from build123d import *

# Parameters (mm, degrees)
F1_DEPTH       = 40
F2_START       = 34
F2_DEPTH       = 6
F3_DEPTH       = 6
F5_D           = 5
F5_DEPTH       = 8
F5_CSINK_D     = 6
F5_CSINK_ANGLE = 90
F5_TIP         = 1.5021515476
F7_D           = 10
F8_D           = 5
F9_SIZE        = 4
F11_D          = 10
F12_R          = 10
F13_D          = 5
F15_D          = 5
F15_DEPTH      = 12
F15_TIP        = 1.5021515476
F16_START      = -7
F14_R          = 5.5
F16_DEPTH      = 5
F17_DEPTH      = 3


with BuildPart() as f1:
    # F0 (on Top) → F1 (new body)
    with BuildSketch(Plane.XY):
        with BuildLine():
            Line((-8.2927711273, 81.5647094006), (-7.3107365454, 75.6475586596))
            ThreePointArc((-7.3107365454, 75.6475586596), (-6.1560843706, 75.7502648525), (-5, 75.8353479586))
            Line((-5, 75.8353479586), (-5, 81.8325844183))
            ThreePointArc((-5, 81.8325844183), (-6.6477349765, 81.7152341505), (-8.2927711273, 81.5647094006))
        make_face()
        with BuildLine():
            Line((-5, 81.8325844183), (-5, 75.8353479586))
            ThreePointArc((-5, 75.8353479586), (0, 76), (5, 75.8353479586))
            Line((5, 75.8353479586), (5, 100.8353479586))
            Line((5, 100.8353479586), (-5, 100.8353479586))
            Line((-5, 100.8353479586), (-5, 81.8325844183))
        make_face()
        with BuildLine():
            ThreePointArc((-13, 68.7822651561), (44.6654228683, 53.8980519128), (70, 0))
            ThreePointArc((70, 0), (44.6654228683, -53.8980519128), (-13, -68.7822651561))
            Line((-13, -68.7822651561), (-13, -74.8799038461))
            ThreePointArc((-13, -74.8799038461), (0, -76), (13, -74.8799038461))
            ThreePointArc((13, -74.8799038461), (18.0414231151, -73.8275494107), (23, -72.4361788059))
            ThreePointArc((23, -72.4361788059), (61.3351449008, -44.8776113446), (76, 0))
            ThreePointArc((76, 0), (55.4797260267, 51.9422756529), (5, 75.8353479586))
            ThreePointArc((5, 75.8353479586), (0, 76), (-5, 75.8353479586))
            ThreePointArc((-5, 75.8353479586), (-6.1560843706, 75.7502648525), (-7.3107365454, 75.6475586596))
            ThreePointArc((-7.3107365454, 75.6475586596), (-9.056731807, 71.7723085764), (-13, 70.1858979679))
            Line((-13, 70.1858979679), (-13, 68.7822651561))
        make_face()
        with BuildLine():
            ThreePointArc((13, -74.8799038461), (0, -76), (-13, -74.8799038461))
            Line((-13, -74.8799038461), (-13, -80.8799038461))
            Line((-13, -80.8799038461), (13, -80.8799038461))
            Line((13, -80.8799038461), (13, -74.8799038461))
        make_face()
        with BuildLine():
            ThreePointArc((23, -72.4361788059), (18.0414231151, -73.8275494107), (13, -74.8799038461))
            Line((13, -74.8799038461), (13, -80.8799038461))
            Line((13, -80.8799038461), (13, -126.8799038461))
            Line((13, -126.8799038461), (23, -126.8799038461))
            Line((23, -126.8799038461), (23, -72.4361788059))
        make_face()
    extrude(amount=F1_DEPTH)

    # F0 (on Top) → F2 (join)
    with BuildSketch(Plane.XY.offset(F2_START)):
        with BuildLine():
            ThreePointArc((-8.009195615, 75.576800578), (-7.6600477823, 75.6129861067), (-7.3107365454, 75.6475586596))
            Line((-7.3107365454, 75.6475586596), (-8.2927711273, 81.5647094006))
            ThreePointArc((-8.2927711273, 81.5647094006), (-11.0489742273, 81.2372577153), (-13.7925136268, 80.8166965449))
            ThreePointArc((-13.7925136268, 80.8166965449), (-9.7567430054, 79.6853320831), (-8, 75.8799038461))
            ThreePointArc((-8, 75.8799038461), (-8.0022994325, 75.7282824834), (-8.009195615, 75.576800578))
        make_face()
        with BuildLine():
            Line((-13, 74.8799038461), (-13, 70.8799038461))
            ThreePointArc((-13, 70.8799038461), (-9.5733045321, 72.2387833907), (-8.009195615, 75.576800578))
            ThreePointArc((-8.009195615, 75.576800578), (-10.5103754149, 75.2697283683), (-13, 74.8799038461))
        make_face()
        with BuildLine():
            ThreePointArc((-17.6052855561, 73.9327662169), (-15.7626356848, 71.7124293023), (-13, 70.8799038461))
            Line((-13, 70.8799038461), (-13, 74.8799038461))
            ThreePointArc((-13, 74.8799038461), (-15.3099687594, 74.441956292), (-17.6052855561, 73.9327662169))
        make_face()
        with BuildLine():
            ThreePointArc((-13.8960239837, 80.7989628029), (-17.3991209977, 78.2564001006), (-17.6052855561, 73.9327662169))
            ThreePointArc((-17.6052855561, 73.9327662169), (-15.3099687594, 74.441956292), (-13, 74.8799038461))
            ThreePointArc((-13, 74.8799038461), (-10.5103754149, 75.2697283683), (-8.009195615, 75.576800578))
            ThreePointArc((-8.009195615, 75.576800578), (-8.0022994325, 75.7282824834), (-8, 75.8799038461))
            ThreePointArc((-8, 75.8799038461), (-9.7567430054, 79.6853320831), (-13.7925136268, 80.8166965449))
            ThreePointArc((-13.7925136268, 80.8166965449), (-13.8442716447, 80.8078462478), (-13.8960239837, 80.7989628029))
        make_face()
        with BuildLine():
            Line((-13, 70.8799038461), (-13, 70.1858979679))
            ThreePointArc((-13, 70.1858979679), (-9.056731807, 71.7723085764), (-7.3107365454, 75.6475586596))
            ThreePointArc((-7.3107365454, 75.6475586596), (-7.6600477823, 75.6129861067), (-8.009195615, 75.576800578))
            ThreePointArc((-8.009195615, 75.576800578), (-9.5733045321, 72.2387833907), (-13, 70.8799038461))
        make_face()
    extrude(amount=F2_DEPTH)

    # F0 (on Top) → F3 (join)
    with BuildSketch(Plane.XY):
        with BuildLine():
            ThreePointArc((-8.009195615, 75.576800578), (-7.6600477823, 75.6129861067), (-7.3107365454, 75.6475586596))
            Line((-7.3107365454, 75.6475586596), (-8.2927711273, 81.5647094006))
            ThreePointArc((-8.2927711273, 81.5647094006), (-11.0489742273, 81.2372577153), (-13.7925136268, 80.8166965449))
            ThreePointArc((-13.7925136268, 80.8166965449), (-9.7567430054, 79.6853320831), (-8, 75.8799038461))
            ThreePointArc((-8, 75.8799038461), (-8.0022994325, 75.7282824834), (-8.009195615, 75.576800578))
        make_face()
        with BuildLine():
            Line((-13, 74.8799038461), (-13, 70.8799038461))
            ThreePointArc((-13, 70.8799038461), (-9.5733045321, 72.2387833907), (-8.009195615, 75.576800578))
            ThreePointArc((-8.009195615, 75.576800578), (-10.5103754149, 75.2697283683), (-13, 74.8799038461))
        make_face()
        with BuildLine():
            ThreePointArc((-17.6052855561, 73.9327662169), (-15.7626356848, 71.7124293023), (-13, 70.8799038461))
            Line((-13, 70.8799038461), (-13, 74.8799038461))
            ThreePointArc((-13, 74.8799038461), (-15.3099687594, 74.441956292), (-17.6052855561, 73.9327662169))
        make_face()
        with BuildLine():
            ThreePointArc((-13.8960239837, 80.7989628029), (-17.3991209977, 78.2564001006), (-17.6052855561, 73.9327662169))
            ThreePointArc((-17.6052855561, 73.9327662169), (-15.3099687594, 74.441956292), (-13, 74.8799038461))
            ThreePointArc((-13, 74.8799038461), (-10.5103754149, 75.2697283683), (-8.009195615, 75.576800578))
            ThreePointArc((-8.009195615, 75.576800578), (-8.0022994325, 75.7282824834), (-8, 75.8799038461))
            ThreePointArc((-8, 75.8799038461), (-9.7567430054, 79.6853320831), (-13.7925136268, 80.8166965449))
            ThreePointArc((-13.7925136268, 80.8166965449), (-13.8442716447, 80.8078462478), (-13.8960239837, 80.7989628029))
        make_face()
        with BuildLine():
            Line((-13, 70.8799038461), (-13, 70.1858979679))
            ThreePointArc((-13, 70.1858979679), (-9.056731807, 71.7723085764), (-7.3107365454, 75.6475586596))
            ThreePointArc((-7.3107365454, 75.6475586596), (-7.6600477823, 75.6129861067), (-8.009195615, 75.576800578))
            ThreePointArc((-8.009195615, 75.576800578), (-9.5733045321, 72.2387833907), (-13, 70.8799038461))
        make_face()
    extrude(amount=F3_DEPTH)

    # F5
    with Locations(Plane(origin=(-13, 0, 0), x_dir=(0, -1, 0), z_dir=(-1, 0, 0))):
        with Locations((74.7822651561, 30), (74.7822651561, 10)):
            CounterSinkHole(F5_D / 2, F5_CSINK_D / 2, depth=F5_DEPTH, counter_sink_angle=F5_CSINK_ANGLE)
            with Locations((0, 0, -(F5_DEPTH + F5_TIP / 2))):  # 118° drill point
                Cone(0, F5_D / 2, F5_TIP, mode=Mode.SUBTRACT)

    # F7 (through all)
    with Locations(Plane.YZ.offset(23)):
        with Locations((-106.8799038461, 20)):
            Hole(F7_D / 2)

    # F8 (through all)
    with Locations(Plane.YZ.offset(23)):
        with Locations((-116.8799038461, 30), (-91.8799038461, 30), (-91.8799038461, 10), (-116.8799038461, 10)):
            Hole(F8_D / 2)

    # F9
    f9_edges = [f1.edges().sort_by_distance(p)[0] for p in [
        (23, -126.879904, 20),
    ]]
    chamfer(f9_edges, length=F9_SIZE)

    # F11 (through all)
    with Locations(Plane.YZ.offset(5)):
        with Locations((90.8353479586, 20)):
            Hole(F11_D / 2)

    # F12
    f12_edges = [f1.edges().sort_by_distance(p)[0] for p in [
        (0, 100.835348, 40),
        (0, 100.835348, 0),
    ]]
    fillet(f12_edges, radius=F12_R)

    # F13 (through all)
    with Locations(Plane(origin=(0, 0, 0), x_dir=(1, 0, 0), z_dir=(0, 0, -1))):
        with Locations((-13, -75.8799038461)):
            Hole(F13_D / 2)

    # F15
    with Locations(Plane.XZ.offset(80.8799038461)):
        with Locations((0, 20)):
            Hole(F15_D / 2, depth=F15_DEPTH)
            with Locations((0, 0, -(F15_DEPTH + F15_TIP / 2))):  # 118° drill point
                Cone(0, F15_D / 2, F15_TIP, mode=Mode.SUBTRACT)

    # F14 (on face) → F16 (cut)
    with BuildSketch(Plane.XZ.offset(80.8799038461).offset(F16_START)):
        with Locations((0, 20)):
            Circle(F14_R)
    extrude(amount=-F16_DEPTH, mode=Mode.SUBTRACT)

    # F6 (on face) → F17 (cut)
    with BuildSketch(Plane.YZ.offset(23)):
        Polygon((-114.5705027693, 34), (-119.1893049229, 34), (-121.4987059996, 30), (-119.1893049229, 26), (-114.5705027693, 26), (-112.2611016926, 30), align=None)
        Polygon((-89.5705027693, 34), (-94.1893049229, 34), (-96.4987059996, 30), (-94.1893049229, 26), (-89.5705027693, 26), (-87.2611016926, 30), align=None)
        Polygon((-87.2611016926, 10), (-89.5705027693, 14), (-94.1893049229, 14), (-96.4987059996, 10), (-94.1893049229, 6), (-89.5705027693, 6), align=None)
        Polygon((-119.1893049229, 14), (-121.4987059996, 10), (-119.1893049229, 6), (-114.5705027693, 6), (-112.2611016926, 10), (-114.5705027693, 14), align=None)
    extrude(amount=-F17_DEPTH, mode=Mode.SUBTRACT)


solid = f1.part
Build history of the part. All positions in model axes, mm. A direction names the side the tool comes from. Give positions to 0.01 mm unless a question says otherwise; leave off trailing zeros. Loops run counter-clockwise (first coordinate to the right, second up) from the corner with the lowest first, then second, coordinate; pieces in that order, holes last. Notation, with made-up numbers: (50, -39.5) - (76, -39.5) arc R23 ccw to (76, -10.5) - close; hole circle Ø8 at (59.25, 74.5). An arc over 180 degrees is marked (long way). Write item = value, one per line. Start each with the question number.
1) Probe probe 1 along Y at (x, z) = (-9.5, 31); probe 2 along X at (y, z) = (-100.5, 31.5); probe 3 along Y at (x, z) = (19, 35.5). List the from-to ranges inside material, lowest first. Write a range as from..to.
2) Pull direction X, two halves, no side cores. Call faces 1 (the flat face through (-3, -73.88, 20)), 2 (the flat face through (23, -98, 20)), 3 (the cylindrical face through (17.93, -109.187, 15.564)): +X half, -X half, draft (parallel to the pull), parting line (faces both ways), or undercut.
3) Band-saw the part on D-D on y = 0. Give the cut face in (x, z), plus the area to 3 significant figures.
4) Band-saw the part on B-B on z = 20. Count the separate pieces of the cut face and the enclosed holes in it, plus the area to 3 significant figures.
5) Band-saw the part on C-C on x = 56. Give the cut face in (y, z).
6) Tool access for faces 4 (the flat face through (-5, 94, 15)), 5 (the flat face through (-7.8, 78.6, 19.8)), 6 (the cylindrical face through (-0.716, -71.86, 25.453)), 7 (the flat face through (5, 85, 20)), 8 (the flat face through (20, -115, 12)): list every direction of +Z, -Z, +X, -X, +Y, -Y with a clear straight run to the whole face (end or side of a thin tool).
7) Band-saw the part on A-A on x = 0. Give the cut face in (y, z), plus the area to 3 significant figures.
8) Drop flat-ended pins along their axis: pin 1 Ø0.9 at (x, y) = (21, -117.5) entering from -Z; pin 2 Ø21 at (y, z) = (88.5, 25) entering from -X; pin 3 Ø12 at (y, z) = (-112.5, 16) entering from -X; pin 4 Ø20 at (y, z) = (89, 18) entering from +X. Give the stop position or say it passes through.
Final values:
q1.probe_1 = -80.88..-77.07, -72.49..-69.35, 69.35..71.39
q1.probe_2 = 13..23
q1.probe_3 = -126.88..-67.37, 67.37..73.59
q2.face_1 = undercut
q2.face_2 = +X half
q2.face_3 = draft
q3.outline = (70, 0) - (76, 0) - (76, 40) - (70, 40) - close
q3.area = 240 mm²
q4.separate_pieces = 4
q4.enclosed_holes = 0
q4.area = 2,160 mm²
q5.outline = (-51.38, 0) - (-42, 0) - (-42, 40) - (-51.38, 40) - close; (42, 0) - (51.38, 0) - (51.38, 40) - (42, 40) - close
q6.face_4 = +Z, -Z, -X, +Y
q6.face_5 = -X
q6.face_6 = none
q6.face_7 = +Z, -Z, +X, +Y
q6.face_8 = +X
q7.outline = (-80.88, 0) - (-70, 0) - (-70, 14.5) - (-73.88, 14.5) - (-73.88, 17.5) - (-80.88, 17.5) - close; (-80.88, 22.5) - (-73.88, 22.5) - (-73.88, 25.5) - (-70, 25.5) - (-70, 40) - (-80.88, 40) - close; (70, 0) - (90.84, 0) arc R10 ccw to (100.84, 10) - (100.84, 30) arc R10 ccw to (90.84, 40) - (70, 40) - close; hole circle Ø10 at (90.84, 20)
q7.area = 1,470 mm²
q8.pin_1 = 0
q8.pin_2 = -8.29
q8.pin_3 = 13
q8.pin_4 = 5
